Geometry: final body of the model. Coordinates: model frame, mm. Give positions to 0.01 mm unless a question says otherwise; leave off trailing zeros. Write each loop counter-clockwise with the first axis right and the second up, starting at its lowest first coordinate (ties: lowest second). Pieces come first, ordered by that corner, then holes. Notation, with made-up numbers: (84.25, 2) -> (112.25, 2) arc R25 ccw to (112.25, 25) -> close; hole circle Ø1 at (79.5, 0.25). An arc over 180 degrees is marked (long way). Use CSV: the item, a comma, the result in double quotes. Start each with the question number.
1) Section C-C (y = 51.5). Output: boundary loops of the cut face in (x, z), plus the area to 3 significant figures.
2) Draft query along X for faces 1 (the face through (-0.17, 149.32, 1.26)), 2 (the face through (1, 68, 0)), 3 (the face through (-0.17, 137.32, 1.26)), 4 (the face through (0, 152, 1)). Return one class per face: pulls with the +X half, pulls with the -X half, needs draft (parallel to the pull), parting line crosses it, or undercut.
3) Section B-B (z = 0.7). Output: boundary loops of the cut face in (x, y), plus the area to 3 significant figures.
4) Section A-A (y = 0). Output: boundary loops of the cut face in (x, z), plus the area to 3 significant figures.
5) Contact query for flat-ended pins moving along their axis: P1, Ø3.5, axis at x = 0, y = 136, coming from the -Z side; P2, Ø1.3, axis at y = 59, z = 1, coming from the +X side; P3, Ø0.8, axis at y = -12.5, z = 1, coming from the -X side; P4, Ø1.6, axis at x = 0, y = 142, coming from the +Z side. Output: stop coordinate, or through.
6) Material intervals for line 1 (X direction, y = 142, z = 1.2); line 2 (X direction, y = 122.5, z = 2.05); line 3 (X direction, y = -1.5, z = 1), sorted ascending. Write a range as [from, to].
```python
from build123d import *

# Parameters (mm, degrees)
MODEL_R             = 3.55
MODEL_R_2           = 1.33
BOSS_EXTRUDE1_DEPTH = 2.55


with BuildPart() as part:
    # Model → Boss-Extrude1 (new body)
    with BuildSketch(Plane.XY):
        with BuildLine():
            Line((-4, 148), (-4, 7.745966692))
            ThreePointArc((-4, 7.745966692), (-4.317541634, 5.245966692), (-5.25, 2.90473751))
            ThreePointArc((-5.25, 2.90473751), (-6, 0), (-5.25, -2.90473751))
            ThreePointArc((-5.25, -2.90473751), (-4.317541634, -5.245966692), (-4, -7.745966692))
            Line((-4, -7.745966692), (-4, -13.8))
            ThreePointArc((-4, -13.8), (0, -17.8), (4, -13.8))
            Line((4, -13.8), (4, -7.745966692))
            ThreePointArc((4, -7.745966692), (4.317541634, -5.245966692), (5.25, -2.90473751))
            ThreePointArc((5.25, -2.90473751), (6, 0), (5.25, 2.90473751))
            ThreePointArc((5.25, 2.90473751), (4.317541634, 5.245966692), (4, 7.745966692))
            Line((4, 7.745966692), (4, 148))
            ThreePointArc((4, 148), (0, 152), (-4, 148))
        make_face()
        Circle(MODEL_R, mode=Mode.SUBTRACT)
        with Locations((0, 148)):
            Circle(MODEL_R_2, mode=Mode.SUBTRACT)
        with Locations((0, 142)):
            Circle(MODEL_R_2, mode=Mode.SUBTRACT)
        with Locations((0, 136)):
            Circle(MODEL_R_2, mode=Mode.SUBTRACT)
        with Locations((0, 130)):
            Circle(MODEL_R_2, mode=Mode.SUBTRACT)
        with BuildLine():
            Line((-1, -10.1), (-1, -13.8))
            ThreePointArc((-1, -13.8), (0, -14.8), (1, -13.8))
            Line((1, -13.8), (1, -10.1))
            ThreePointArc((1, -10.1), (0, -9.1), (-1, -10.1))
        make_face(mode=Mode.SUBTRACT)
        with BuildLine():
            Line((-1, 15.1), (-1, 10.1))
            ThreePointArc((-1, 10.1), (0, 9.1), (1, 10.1))
            Line((1, 10.1), (1, 15.1))
            ThreePointArc((1, 15.1), (0, 16.1), (-1, 15.1))
        make_face(mode=Mode.SUBTRACT)
    extrude(amount=BOSS_EXTRUDE1_DEPTH)


solid = part.part
```
Answers follow:
1,outline,"(-4, 0) -> (4, 0) -> (4, 2.55) -> (-4, 2.55) -> close"
1,area,"20.4 mm^2"
2,face 1,"undercut"
2,face 2,"needs draft"
2,face 3,"undercut"
2,face 4,"parting line crosses it"
3,outline,"(-5.25, -2.9) arc R10 cw to (-4, -7.75) -> (-4, -13.8) arc R4 ccw to (4, -13.8) -> (4, -7.75) arc R10 cw to (5.25, -2.9) arc R6 ccw to (5.25, 2.9) arc R10 cw to (4, 7.75) -> (4, 148) arc R4 ccw to (-4, 148) -> (-4, 7.75) arc R10 cw to (-5.25, 2.9) arc R6 ccw to start; hole circle Ø7.1 at (0, 0); hole circle Ø2.66 at (0, 130); hole circle Ø2.66 at (0, 136); hole circle Ø2.66 at (0, 142); hole circle Ø2.66 at (0, 148); hole (-1, -13.8) arc R1 ccw to (1, -13.8) -> (1, -10.1) arc R1 ccw to (-1, -10.1) -> close; hole (-1, 10.1) arc R1 ccw to (1, 10.1) -> (1, 15.1) arc R1 ccw to (-1, 15.1) -> close"
3,area,"1,290 mm^2"
4,outline,"(-6, 0) -> (-3.55, 0) -> (-3.55, 2.55) -> (-6, 2.55) -> close; (3.55, 0) -> (6, 0) -> (6, 2.55) -> (3.55, 2.55) -> close"
4,area,"12.5 mm^2"
5,P1,"stops at z = 0"
5,P2,"stops at x = 4"
5,P3,"stops at x = -4"
5,P4,"passes through"
6,line 1,"x = [-4, -1.33], [1.33, 4]"
6,line 2,"x = [-4, 4]"
6,line 3,"x = [-5.81, -3.22], [3.22, 5.81]"
